Geometry: see drawing. Coordinates: mm, zero at the bounding-box minimum. A direction names the side the tool comes from. Give positions to 0.01 mm unless a question says otherwise; leave off trailing zeros. Write each loop counter-clockwise with the first axis right and the second up, starting at its lowest first coordinate (ties: lowest second). Pieces come first, ordered by that corner, then holes. Notation, with made-up numbers: (-32.75, 33) -> (16.25, 33) arc R20 cw to (16.25, 52) -> close; hole circle Ø6 at (77, 26). An arc over 180 degrees is marked (long way). Answer as a JSON object with one key per item and string values. Group by question number.
Item 1: Access query for the marked faces 1, 2 and 3. Directions: +Z, -Z, +X, -X, +Y, -Y. A direction counts if a zero-diameter tool reaches every point of the face in a straight line with its end or side. Return the directions, or none.
Item 2: Section query C-C on x = 1.54. Return the cut outline in (y, z), plus the area to 3 significant figures.
Item 3: Section query D-D on y = 0.55. Return the cut outline in (x, z).
Item 4: Section query B-B on y = 4.3. Return the cut outline in (x, z).
Item 5: Section query A-A on z = 6. Return the cut outline in (x, y).
Item 6: First-contact query: pin 1 Ø2.5 at (x, z) = (5.5, 5) entering from -Y; pin 2 Ø1.4 at (x, y) = (5, 3.5) entering from +Z. Flat tips, straight axial feed; report the tip coordinate or a pass-through.
Item 7: Ray query, probe 1 along Y at (x, z) = (4.75, 7.25); probe 2 along X at (y, z) = (3.2, 5.5); probe 3 along Y at (x, z) = (9.5, 7.25) (1 decimal). Return the intervals inside material, ascending. Write a range as from..to.
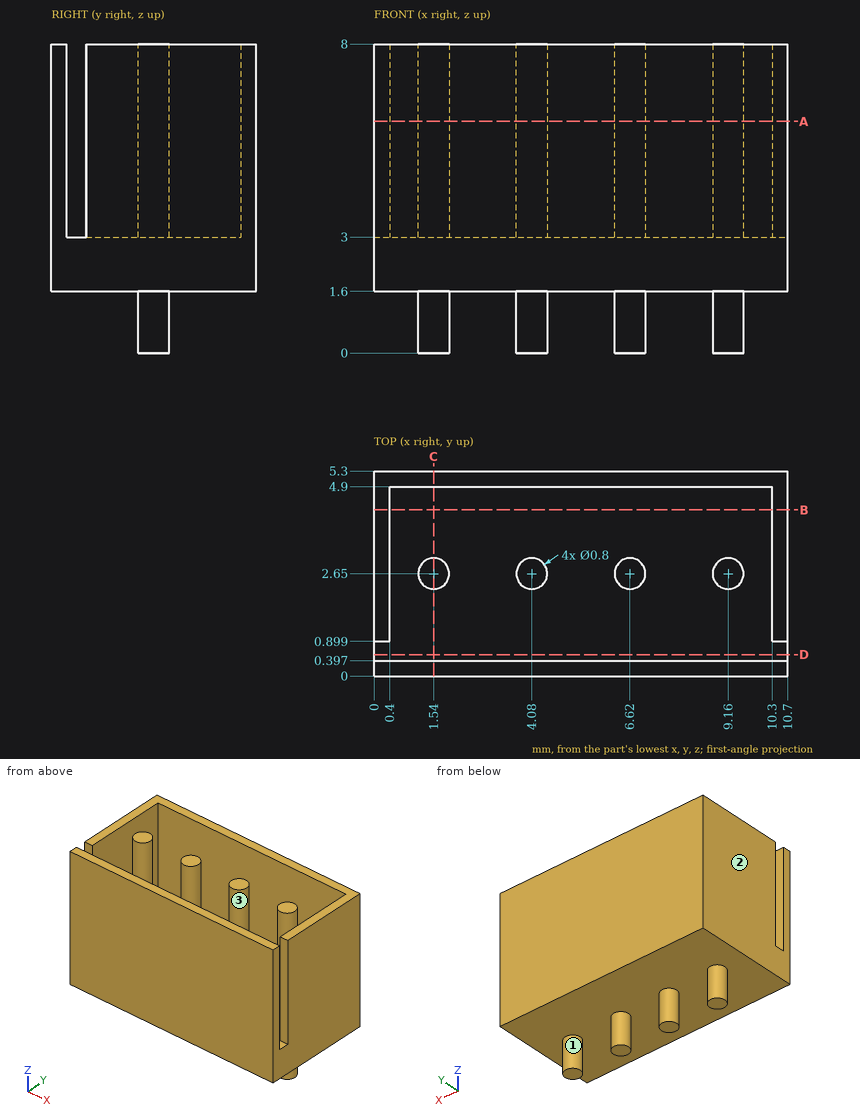
Worked answers:
{
 "1": {"face 1": "-Z", "face 2": "+Z, -Z, -X, +Y, -Y", "face 3": "+Z"},
 "2": {"outline": "(0, 1.6) -> (2.25, 1.6) -> (2.25, 0) -> (3.05, 0) -> (3.05, 1.6) -> (5.3, 1.6) -> (5.3, 8) -> (4.9, 8) -> (4.9, 3) -> (3.05, 3) -> (3.05, 8) -> (2.25, 8) -> (2.25, 3) -> (0.4, 3) -> (0.4, 8) -> (0, 8) -> close", "area": "16.7 mm^2"},
 "3": {"outline": "(0, 1.6) -> (10.7, 1.6) -> (10.7, 3) -> (0, 3) -> close"},
 "4": {"outline": "(0, 1.6) -> (10.7, 1.6) -> (10.7, 8) -> (10.3, 8) -> (10.3, 3) -> (0.4, 3) -> (0.4, 8) -> (0, 8) -> close"},
 "5": {"outline": "(0, 0) -> (10.7, 0) -> (10.7, 0.4) -> (0, 0.4) -> close; (0, 0.9) -> (0.4, 0.9) -> (0.4, 4.9) -> (10.3, 4.9) -> (10.3, 0.9) -> (10.7, 0.9) -> (10.7, 5.3) -> (0, 5.3) -> close; circle Ø0.8 at (1.54, 2.65); circle Ø0.8 at (4.08, 2.65); circle Ø0.8 at (6.62, 2.65); circle Ø0.8 at (9.16, 2.65)"},
 "6": {"pin 1": "y = 0", "pin 2": "z = 3"},
 "7": {"probe 1": "0..0.4, 4.9..5.3", "probe 2": "0..0.4, 10.3..10.7", "probe 3": "0..0.4, 2.4..2.9, 4.9..5.3"}
}
